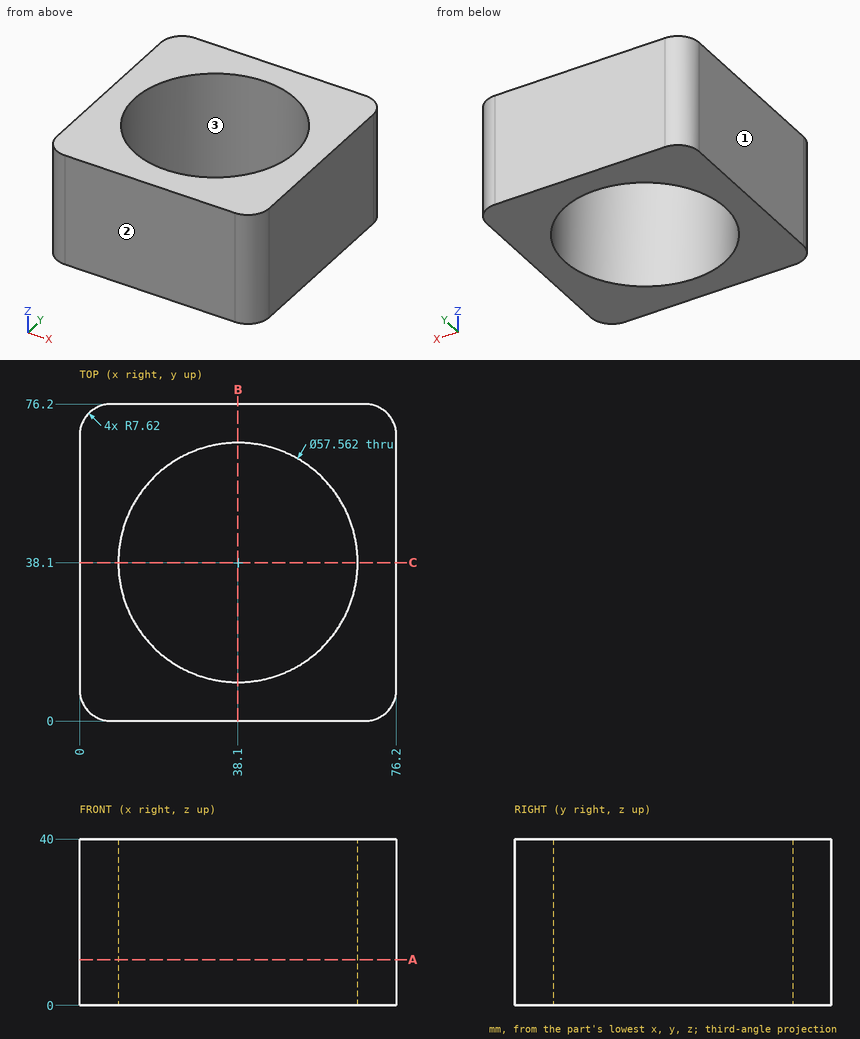
The drawing under review shows one solid part. Ordinate dimensions are in mm from its lowest x, y, z. Coordinates: 2 decimals unless noted, no trailing zeros. Loops run counter-clockwise (first coordinate to the right, second up) from the corner with the lowest first, then second, coordinate; pieces in that order, holes last. Notation, with made-up numbers: M -13.75,30 L 39.25,30 A29 ccw 39.25,53 Z; hole C 76,68 d10. An arc over 180 degrees is marked long. Use one line per item in the form item = value.
(1) Consider section B-B (x = 38.1). Write out the cut boundary in (y, z), and give its area (3 significant figures).
Return value:
outline = M 0,0 L 9.32,0 L 9.32,40 L 0,40 Z; M 66.88,0 L 76.2,0 L 76.2,40 L 66.88,40 Z
area = 746 mm2
(2) Consider section A-A (z = 11). Write out the cut boundary in (x, y).
Return value:
outline = M 0,7.62 A7.62 ccw 7.62,0 L 68.58,0 A7.62 ccw 76.2,7.62 L 76.2,68.58 A7.62 ccw 68.58,76.2 L 7.62,76.2 A7.62 ccw 0,68.58 Z; hole C 38.1,38.1 d57.56
(3) For line 1 along X through (y, z) = (37, 22); line 2 along X through (y, z) = (50, 37); line 3 along Y through (x, z) = (18, 24), list the stretches that pass through material, from the lowest coordinate up. Write a range as from..to.
Return value:
line_1 = 0..9.34, 66.86..76.2
line_2 = 0..11.89, 64.31..76.2
line_3 = 0..17.5, 58.7..76.2
(4) Clearance check with a flat-ended pin moving along its axis: P1, Ø6, axis at x = 46.5, y = 15.5, coming from the +Z side. State where the tip first meets the part, or that it passes through.
Return value:
P1 = through
(5) Draft analysis for pull direction Y (two halves, no side actions). For the marked faces 1, 2 and 3, state which applies: pulls with the +Y half, pulls with the -Y half, needs draft (parallel to the pull), parting line crosses it, or undercut.
Return value:
face_1 = needs draft
face_2 = pulls with the -Y half
face_3 = undercut
